Check sheet for the modelled part. Datum: model origin and axes. Units: mm. Give positions to 0.01 mm unless a question says otherwise; leave off trailing zeros. Loops run counter-clockwise (first coordinate to the right, second up) from the corner with the lowest first, then second, coordinate; pieces in that order, holes last. Notation, with made-up numbers: (26, 32.25) -> (40, 32.25) arc R28 ccw to (40, 50.25) -> close; hole circle Ø5 at (46.25, -0.75). An arc over 180 degrees is marked (long way). Write each question's results on one line, items separated by ' | '. Start each with the question number.
Item 1: Cross-section at A-A on y = 0. Enter the section's corners in (x, z).
Item 2: Mould release check, pull along Y, two halves, no side actions. Record for faces 1 (the face through (-69.178, -28.763, 7.605)), 2 (the face through (-99.257, -23, 7)), 3 (the face through (-1, 27.7, 7)): pulls with the +Y half, pulls with the -Y half, needs draft (parallel to the pull), parting line crosses it, or undercut.
Item 3: Scan lines: line 1 along X through (y, z) = (-2, 5); line 2 along X through (y, z) = (6, 1.25); line 3 along Y through (x, z) = (81, 4.75). Record each from-to range of solid material in increasing order.
Item 4: Cross-section at C-C on z = 3.5. Enter the section's corners in (x, y), then the cut area to 3 significant figures.
Item 5: Cross-section at B-B on x = 70. Enter the section's corners in (y, z).
Item 6: Cross-section at D-D on y = -42. Enter the section's corners in (x, z).
from build123d import *

# Parameters (mm, degrees)
F0_W     = 200
F0_H     = 100
F1_DEPTH = 15
F2_R     = 15
F3_DEPTH = 15.001
F4_R     = 15.498481
F5_DEPTH = 15.001
F6_DEPTH = 15.001


with BuildPart() as f1:
    # F0 (on Top) → F1 (new body)
    with BuildSketch(Plane.XY):
        with Locations((0.742927, -22.300308)):
            Rectangle(F0_W, F0_H)
    extrude(amount=F1_DEPTH)

    # F2 (on face) → F3 (cut, through all)
    with BuildSketch(Plane.XY.offset(15)):
        with Locations((-67.708292, 0)):
            Circle(F2_R)
        with Locations((3.691708, 0)):
            Circle(F2_R)
        with Locations((75.091708, 0)):
            Circle(F2_R)
    extrude(amount=-F3_DEPTH, mode=Mode.SUBTRACT)

    # F4 (on face) → F5 (cut, through all)
    with BuildSketch(Plane.XY.offset(15)):
        with Locations((-67.160375, -44.129718)):
            Circle(F4_R)
    extrude(amount=-F5_DEPTH, mode=Mode.SUBTRACT)

    # F4 (on face) → F6 (cut, through all)
    with BuildSketch(Plane.XY.offset(15)):
        with Locations((-67.160375, -44.129718)):
            Circle(F4_R)
        with Locations((3.639625, -44.129718)):
            Circle(F4_R)
        with Locations((74.439625, -44.129718)):
            Circle(F4_R)
    extrude(amount=-F6_DEPTH, mode=Mode.SUBTRACT)


solid = f1.part
Answer sheet:
1) outline: (-99.26, 0) -> (-82.71, 0) -> (-82.71, 15) -> (-99.26, 15) -> close; (-52.71, 0) -> (-11.31, 0) -> (-11.31, 15) -> (-52.71, 15) -> close; (18.69, 0) -> (60.09, 0) -> (60.09, 15) -> (18.69, 15) -> close; (90.09, 0) -> (100.74, 0) -> (100.74, 15) -> (90.09, 15) -> close
2) face 1: undercut | face 2: needs draft | face 3: pulls with the +Y half
3) line 1: x = -99.26 to -82.57, -52.84 to -11.17, 18.56 to 60.23, 89.96 to 100.74 | line 2: x = -99.26 to -81.46, -53.96 to -10.06, 17.44 to 61.34, 88.84 to 100.74 | line 3: y = -72.3 to -58.17, -30.09 to -13.79, 13.79 to 27.7
4) outline: (-99.26, -72.3) -> (100.74, -72.3) -> (100.74, 27.7) -> (-99.26, 27.7) -> close; hole circle Ø30 at (-67.71, 0); hole circle Ø31 at (-67.16, -44.13); hole circle Ø31 at (3.64, -44.13); hole circle Ø30 at (3.69, 0); hole circle Ø31 at (74.44, -44.13); hole circle Ø30 at (75.09, 0) | area: 15,600 mm²
5) outline: (-72.3, 0) -> (-58.98, 0) -> (-58.98, 15) -> (-72.3, 15) -> close; (-29.28, 0) -> (-14.11, 0) -> (-14.11, 15) -> (-29.28, 15) -> close; (14.11, 0) -> (27.7, 0) -> (27.7, 15) -> (14.11, 15) -> close
6) outline: (-99.26, 0) -> (-82.51, 0) -> (-82.51, 15) -> (-99.26, 15) -> close; (-51.81, 0) -> (-11.71, 0) -> (-11.71, 15) -> (-51.81, 15) -> close; (18.99, 0) -> (59.09, 0) -> (59.09, 15) -> (18.99, 15) -> close; (89.79, 0) -> (100.74, 0) -> (100.74, 15) -> (89.79, 15) -> close
